Read the model definition and answer for the solid it produces. Units are mm, in the model's axes. A direction names the side the tool comes from. Round coordinates to 2 decimals unless told otherwise and drop trailing zeros. Order: outer loops, then holes, each group sorted by start corner. A loop starts at its lowest first (then second) coordinate and runs counter-clockwise, first axis right, second up.
Autodesk Inventor part; units mm, degrees
ref_plane "YZ Plane" through (0, 0, 0) normal (1, 0, 0) x (0, 1, 0)
ref_plane "XZ Plane" through (0, 0, 0) normal (0, 1, 0) x (-1, 0, 0)
ref_plane "XY Plane" through (0, 0, 0) normal (0, 0, 1) x (1, 0, 0)
sketch "Sketch1" plane through (0, 0, 0) normal (0, 1, 0) x (-1, 0, 0)
  line L0 (10, 20) -> (0, 20)
  line L1 (0, 20) -> (0, -20)
  line L2 (0, -20) -> (10, -20)
  line L3 (10, -20) -> (10, 20)
  line L4 (10, 20) -> (3, 20)
  line L5 (3, 20) -> (3, 13)
  line L6 (3, 13) -> (10, 13)
  line L7 (10, 13) -> (10, 20)
  line L8 (10, -20) -> (3, -20)
  line L9 (3, -20) -> (3, -13)
  line L10 (3, -13) -> (10, -13)
  line L11 (10, -13) -> (10, -20)
  point P0 (0, 0)
  point P1 (0, 0)
  dimension "d0" = 10
  dimension "d1" = 40
  dimension "d2" = 7
  dimension "d3" = 7
  dimension "d4" = 7
  dimension "d5" = 7
extrude "Extrusion1" add sketch "Sketch1" along normal blind 20 contours L5 L6 L3 L10 L9 L2 L1 L0
sketch "Sketch2" plane through (-10, 0, -13) normal (-1, 0, 0) x (0, 0, 1)
  line L0 (0, 0) -> (26, 0)
  line L1 (0, 0) -> (0, 20)
  line L2 (26, 0) -> (0, 0)
  line L3 (0, 0) -> (0, 15)
  line L4 (0, 15) -> (26, 15)
  line L5 (26, 15) -> (26, 0)
  circle A0 centre (29.5, 10) radius 2
  circle A1 centre (-3.5, 10) radius 2
  line L6 (-7, 0) -> (-7, 20)
  line L7 (26, 0) -> (33, 0)
  line L8 (-7, 0) -> (0, 0)
  point P0 (13, 0)
  point P1 (-7, 10)
  point P2 (29.5, 0)
  point P3 (-3.5, 0)
  dimension "d8" = 15
  dimension "d9" = 4
  dimension "d10" = 4
extrude "Extrusion2" cut sketch "Sketch2" against normal through all
sketch "Sketch3" plane through (-10, 20, -13) normal (-1, 0, 0) x (0, 0, 1)
  circle A0 centre (20.5, -2.5) radius 1
  circle A1 centre (5.5, -2.5) radius 1
  line L0 (0, -5) -> (0, 0)
  line L1 (20.5, -2.5) -> (5.5, -2.5)
  line L2 (0, -5) -> (26, -5)
  point P0 (13, -20)
  point P1 (0, -2.5)
  point P2 (13, -2.5)
  point P3 (13, -5)
  dimension "d13" = 2
  dimension "d14" = 2
  dimension "d15" = 15
extrude "Extrusion3" cut sketch "Sketch3" against normal through all
fillet "Fillet1" radius 4 4 edges at (-3, 17.5, -13) (-3, 17.5, 13) (-1.5, 15, -13) (-1.5, 15, 13)
fillet "Fillet2" radius 2 4 edges at (-3, 15, 15) (-3, 15, 11) (-3, 15, -15) (-3, 15, -11)
properties part number "mpu6050"
Q1. Straight lines are drawn through the part: probe 1 along Y at (x, z) = (-1, -16.5); probe 2 along Y at (x, z) = (-3.5, 7.5); probe 3 along X at (y, z) = (13, -17). For each, find the intervals that lie inside material, in ascending order.
Outcome:
probe 1: y = 0 to 8, 12 to 20
probe 2: y = 15 to 16.5, 18.5 to 20
probe 3: x = -3 to 0
Q2. For a pull along Y with two mould halves and no side action, classify faces 6 (the face through (-3.6, 14.43, -13.06)), 7 (the face through (-4, 20, 0)), 8 (the face through (-8, 17, 13)), 9 (the face through (-5.07, 16.524, -7.717)) as released by +Y, released by -Y, zero draft, split by the parting line, or undercut.
Outcome:
face 6: released by -Y
face 7: released by +Y
face 8: zero draft
face 9: undercut
Q3. A cutting plane is placed at B-B, the plane y = 10. Give the vertices of the cut face in (x, z).
Outcome:
outline: (-3, -20) - (0, -20) - (0, -18.5) - (-3, -18.5) - close; (-3, -14.5) - (0, -14.5) - (0, -13) - (-3, -13) - close; (-3, 13) - (0, 13) - (0, 14.5) - (-3, 14.5) - close; (-3, 18.5) - (0, 18.5) - (0, 20) - (-3, 20) - close
Q4. A cutting plane is placed at A-A, the plane y = 4. Give the vertices of the cut face in (x, z).
Outcome:
outline: (-3, -20) - (0, -20) - (0, -13) - (-3, -13) - close; (-3, 13) - (0, 13) - (0, 20) - (-3, 20) - close
Q5. For faces 1 (the face through (-10, 17, 0)), 2 (the face through (-3, 7.6, -17.1)), 3 (the face through (-1.91, 14.3, 11.26)), 4 (the face through (-5, 15, 0)), 5 (the face through (-3, 7.6, 17.1)), determine the directions among +Z, -Z, +X, -X, +Y, -Y from which every point of the face is accessible in a straight line to the end or side of a thin tool.
Outcome:
face 1: +Z, -Z, -X, +Y, -Y
face 2: -Z, -X, -Y
face 3: +X, -X, -Y
face 4: -X, -Y
face 5: +Z, -X, -Y
Q6. A cutting plane is placed at D-D, the plane x = -8.5. Give the vertices of the cut face in (y, z), plus the area to 3 significant figures.
Outcome:
outline: (15, -13) - (20, -13) - (20, 13) - (15, 13) - close; hole circle Ø2 at (17.5, -7.5); hole circle Ø2 at (17.5, 7.5)
area: 124 mm2
Q7. A cutting plane is placed at C-C, the plane z = 7.5. Give the vertices of the cut face in (x, y), plus the area to 3 significant figures.
Outcome:
outline: (-10, 15) - (0, 15) - (0, 16.5) - (-10, 16.5) - close; (-10, 18.5) - (0, 18.5) - (0, 20) - (-10, 20) - close
area: 30.0 mm2
Q8. Flat-ended cylindrical pins translate along their axes: pin 1 (2 mm diameter, centred on x = -5.5, z = -6, fed in from -Y); pin 2 (5 mm diameter, centred on x = -6.5, y = 15.5, fed in from +Z); pin 3 (6 mm diameter, centred on y = 8, z = 14.5, fed in from -X). Find the tip coordinate at first contact, or state that the pin passes through.
Outcome:
pin 1: stops at y = 15
pin 2: stops at z = 14.35
pin 3: stops at x = -3
